Could you check a few things on this drawing? It's one solid part, dimensions in mm from its lowest x, y, z. Coordinates: 2 decimals unless noted, no trailing zeros. Loops run counter-clockwise (first coordinate to the right, second up) from the corner with the lowest first, then second, coordinate; pieces in that order, holes last. Notation, with made-up numbers: (80.5, 18.25) -> (125.5, 18.25) arc R28 cw to (125.5, 57.25) -> close; hole circle Ø2 at (83, 71). An arc over 180 degrees is marked (long way). One line per question, with ' | ' between items. Start each with the question number.
(1) I'm going to push flat-ended pins straight in: pin 1 Ø13 at (x, z) = (44.5, 69) entering from -Y; pin 2 Ø2.5 at (y, z) = (7.5, 13) entering from +X; pin 3 Ø5.5 at (x, y) = (13.5, 5.5) entering from +Z. Where does each tip first touch, or does it pass through?
(2) Suppose I cut it at B-B (z = 69). Please give me the cut outline in (x, y) (1 decimal).
(3) If I drill on line 1 along X through (y, z) = (5, 64); line 2 along Y through (x, z) = (21.5, 10.5); line 3 along Z through (x, y) = (11, 10.5) (1 decimal), over which ranges is the centre line in solid material (lowest first)?
(4) Suppose I cut it at A-A (y = 3). Please give me the cut outline in (x, z), plus the area to 3 significant figures.
(5) Suppose I cut it at C-C (x = 40.5). Please give me the cut outline in (y, z), plus the area to 3 significant figures.
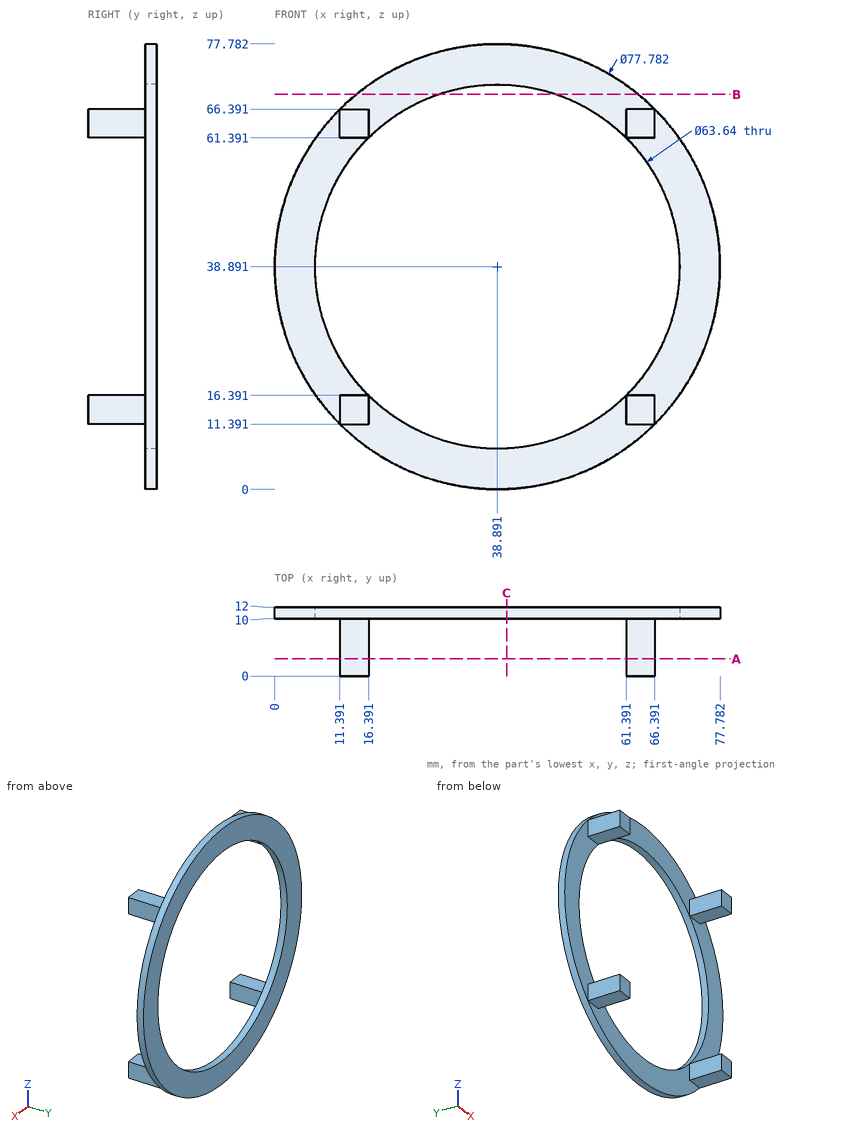
Checks:
1) pin 1: stops at y = 10 | pin 2: stops at x = 66.39 | pin 3: stops at z = 66.39
2) outline: (14.3, 10) -> (28.6, 10) -> (28.6, 12) -> (14.3, 12) -> close; (49.2, 10) -> (63.5, 10) -> (63.5, 12) -> (49.2, 12) -> close
3) line 1: x = 11.39 to 16.39, 61.39 to 66.39 | line 2: y = 10 to 12 | line 3: z = 11.8 to 23.6, 54.2 to 66
4) outline: (11.39, 11.39) -> (16.39, 11.39) -> (16.39, 16.39) -> (11.39, 16.39) -> close; (11.39, 61.39) -> (16.39, 61.39) -> (16.39, 66.39) -> (11.39, 66.39) -> close; (61.39, 11.39) -> (66.39, 11.39) -> (66.39, 16.39) -> (61.39, 16.39) -> close; (61.39, 61.39) -> (66.39, 61.39) -> (66.39, 66.39) -> (61.39, 66.39) -> close | area: 100 mm^2
5) outline: (10, 0.03) -> (12, 0.03) -> (12, 7.11) -> (10, 7.11) -> close; (10, 70.67) -> (12, 70.67) -> (12, 77.75) -> (10, 77.75) -> close | area: 28.3 mm^2
